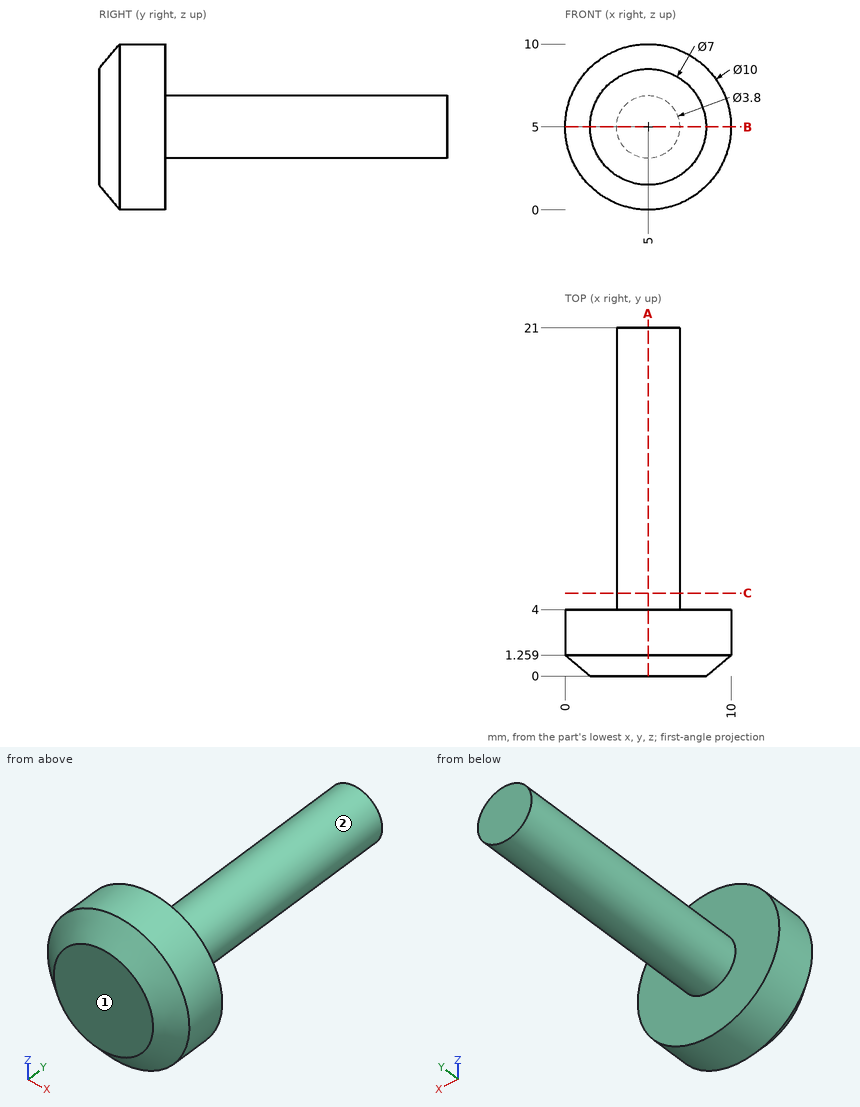
Can you work these out from the drawing? Everything is in mm from the part's minimum corner. A direction names the side the tool comes from. Give positions to 0.01 mm unless a question says otherwise; leave off trailing zeros. Write each loop counter-clockwise with the first axis right and the second up, starting at its lowest first coordinate (ties: lowest second). Pieces come first, ordered by that corner, then holes. Notation, with made-up numbers: M 58.5,-26 L 112.5,-26 A30 cw 112.5,10 Z; hole C -16,-25 d10. An arc over 180 degrees is marked long. Answer in a Markdown table with one row per item. Add a question column.
Item 1: Imagine slicing it at A-A, the plane x = 5. Write out the boundary of the cut face in (y, z), plus the area to 3 significant figures.
Item 2: For pin 1 Ø3 at (x, y) = (7, 11) entering from +Z; pin 2 Ø1 at (y, z) = (13, 7.5) entering from +X; pin 3 Ø2 at (x, y) = (4, 10) entering from +Z; pin 4 Ø1 at (x, z) = (9, 4.5) entering from -Y (1 decimal), each with a flat end and sliding along its axis, tell me the tip position at first contact or that it passes through.
Item 3: Imagine slicing it at B-B, the plane z = 5. Write out the boundary of the cut face in (x, y), plus the area to 3 significant figures.
Item 4: Please list where these lines run through material, in increasing order: L1, parallel to Y at x = 3, z = 7.75; L2, parallel to X at y = 7.5, z = 4.75; L3, parallel to Z at x = 6.5, y = 7.5 (1 decimal).
Item 5: Imagine slicing it at C-C, the plane y = 5. Write out the boundary of the cut face in (x, z).
Item 6: On a 3-axis mill with a long thin cutter (end or side, diameter ignored), from which of +Z, -Z, +X, -X, +Y, -Y can I reach the whole of each face in a straight line? I mean the marked faces 1 and 2. Say none if no direction works.
Evaluation:
| question | item | result |
|---|---|---|
| 1 | outline | M 0,1.5 L 1.26,0 L 4,0 L 4,3.1 L 21,3.1 L 21,6.9 L 4,6.9 L 4,10 L 1.26,10 L 0,8.5 Z |
| 1 | area | 103 mm² |
| 2 | pin 1 | stops at z = 6.83 |
| 2 | pin 2 | passes through |
| 2 | pin 3 | stops at z = 6.9 |
| 2 | pin 4 | stops at y = 0 |
| 3 | outline | M 0,1.26 L 1.5,0 L 8.5,0 L 10,1.26 L 10,4 L 6.9,4 L 6.9,21 L 3.1,21 L 3.1,4 L 0,4 Z |
| 3 | area | 103 mm² |
| 4 | L1 | y = 0 to 4 |
| 4 | L2 | x = 3.12 to 6.88 |
| 4 | L3 | z = 3.8 to 6.2 |
| 5 | outline | C 5,5 d3.8 |
| 6 | face 1 | +Z, -Z, +X, -X, -Y |
| 6 | face 2 | +Y |
